Input: part model. Units: mm. Frame: model coordinates. A direction names the side the tool comes from. Give positions to 0.01 mm unless a question says otherwise; leave off trailing zeros. Order: outer loops, then holes, each group sorted by start corner. A loop starts at its lowest first (then second) coordinate and runs counter-clockwise, first axis right, second up. Notation, with made-up numbers: M 87.25,-25.5 L 104.25,-25.5 A20 cw 104.25,4.5 Z; hole C -12,5 d10. An arc over 180 degrees is marked long. Use a Markdown table: item, result.
Autodesk Fusion 360 part; units mm, degrees
sketch "Sketch1" plane through (0, 0, 0) normal (0, 0, 1) x (1, 0, 0)
  line L0 (-27.5, 5) -> (27.5, 5)
  line L1 (27.5, 5) -> (27.5, -5)
  line L2 (27.5, -5) -> (-27.5, -5)
  line L3 (-27.5, -5) -> (-27.5, 5)
  line L4 (-27.5, 5) -> (27.5, -5) construction
  line L5 (27.5, 5) -> (-27.5, -5) construction
  dimension "d1" = 55
  dimension "d2" = 10
sketch "Sketch2" plane through (0, 0, 0) normal (0, 0, 1) x (1, 0, 0)
  line L0 (-27.5, 0) -> (-20, 0) construction
  line L1 (27.5, 0) -> (20, 0) construction
  dimension "d3" = 7.5
  dimension "d4" = 7.5
sketch "Sketch3" plane through (0, 0, 0) normal (0, 0, 1) x (1, 0, 0)
  circle A0 centre (-20, 0) radius 1.8
  circle A1 centre (20, 0) radius 1.8
  dimension "d7" = 3.6
  dimension "d8" = 3.6
extrude "Extrude1" add sketch "Sketch1" along normal blind 2
extrude "Extrude2" cut sketch "Sketch3" along normal blind 10
sketch "Sketch5" plane through (0, 5, 0) normal (0, 1, 0) x (-1, 0, 0)
  line L0 (-27.5, 0) -> (27.5, 0)
  line L1 (27.5, 0) -> (27.5, 2)
  line L2 (27.5, 2) -> (-27.5, 2)
  line L3 (-27.5, 2) -> (-27.5, 0)
  line L4 (-5, 2) -> (5, 2)
  line L5 (5, 2) -> (5, 0)
  line L6 (5, 0) -> (-5, 0)
  line L7 (-5, 0) -> (-5, 2)
extrude "Extrude3" add sketch "Sketch5" along normal blind 25 contours L0 L2 L4 L5 L6 L7
sketch "Sketch6" plane through (0, 0, 2) normal (0, 0, 1) x (-1, 0, 0)
  circle A0 centre (-20, 0) radius 1.8
  circle A1 centre (20, 0) radius 1.8
  line L0 (27.5, 5) -> (-27.5, 5)
  line L1 (-27.5, 5) -> (-27.5, -5)
  line L2 (-27.5, -5) -> (-5, -5)
  line L3 (-5, -5) -> (-5, -30)
  line L4 (-5, -30) -> (5, -30)
  line L5 (5, -30) -> (5, -5)
  line L6 (5, -5) -> (27.5, -5)
  line L7 (27.5, -5) -> (27.5, 5)
  circle A2 centre (0, -25) radius 4.2426
extrude "Extrude4" add sketch "Sketch6" along normal blind 20 contours A2
fillet "Fillet1" radius 3 1 edges at (3.9555, 26.5342, 22)
fillet "Fillet2" radius 1 1 edges at (3.9555, 23.4658, 2)
chamfer "Chamfer1" distance 1 angle 45 8 edges at (-5, 17.5, 0) (5, 17.5, 0) (0, 30, 0) (-16.25, 5, 0) (-27.5, 0, 0) (0, -5, 0) (27.5, 0, 0) (16.25, 5, 0)
extrude "Extrude5" add 1 faces at (-5, 19.4745, 1.3333) along direction (-1, 0, 0) blind 5
extrude "Extrude6" add 1 faces at (5, 19.4745, 1.3333) along direction (1, 0, 0) blind 5
extrude "Extrude7" add 1 faces at (-0.5255, 30, 1.3333) along direction (0, 1, 0) blind 5
extrude "Extrude8" cut 1 faces at (1.6667, 35, 1.3333) along direction (0, -1, 0) blind 4
1) Material intervals for line 1 (X direction, y = 0, z = 1.2); line 2 (Y direction, x = -20, z = 1.5); line 3 (Z direction, x = -6.5, y = 22.5), sorted ascending. Write a range as from..to.
Response values:
| item | result |
|---|---|
| line 1 | x = -27.5..-21.8, -18.2..18.2, 21.8..27.5 |
| line 2 | y = -5..-1.8, 1.8..5 |
| line 3 | z = 1..2 |
2) Reachability of faces 4 (the face through (0, 25, 22)), 5 (the face through (-7, 18, 1)) from +Z, -Z, +X, -X, +Y, -Y: full face, straight path, thin tool, end or side. Return the list, or none.
Response values:
| item | result |
|---|---|
| face 4 | +Z, +X, -X, +Y, -Y |
| face 5 | -Z, +Y |
3) Mould query, pull axis Y, two halves, no side actions, for faces 1 (the face through (21.717, -0.541, 0.986)), 2 (the face through (0, 6, 0)), 3 (the face through (3, 22, 11)). Classes: released by +Y, released by -Y, zero draft, split by the parting line, or undercut.
Response values:
| item | result |
|---|---|
| face 1 | undercut |
| face 2 | zero draft |
| face 3 | split by the parting line |
4) Cut plane D-D on y = 14. Return loops of the section in (x, z), and give its area (3 significant figures).
Response values:
| item | result |
|---|---|
| outline | M -10,1 L -5,1 L -4,0 L 4,0 L 5,1 L 10,1 L 10,2 L -10,2 Z |
| area | 29.0 mm² |
5) Cut plane A-A on y = 0. Return loops of the section in (x, z).
Response values:
| item | result |
|---|---|
| outline | M -27.5,1 L -26.5,0 L -21.8,0 L -21.8,2 L -27.5,2 Z; M -18.2,0 L 18.2,0 L 18.2,2 L -18.2,2 Z; M 21.8,0 L 26.5,0 L 27.5,1 L 27.5,2 L 21.8,2 Z |
6) Cut plane B-B on x = 20. Return loops of the section in (y, z).
Response values:
| item | result |
|---|---|
| outline | M -5,1 L -4,0 L -1.8,0 L -1.8,2 L -5,2 Z; M 1.8,0 L 4,0 L 5,1 L 5,2 L 1.8,2 Z |
7) Cut plane C-C on x = 9. Return loops of the section in (y, z).
Response values:
| item | result |
|---|---|
| outline | M -5,1 L -4,0 L 4,0 L 5,1 L 31,1 L 31,2 L -5,2 Z |
8) First-contact query: pin 1 Ø1.1 at (y, z) = (24.5, 1.5) entering from -X; pin 2 Ø0.8 at (x, z) = (15, 1.5) entering from +Y; pin 3 Ø1 at (x, y) = (9, 19) entering from +Z; pin 4 Ø8 at (x, z) = (21.5, 9.5) entering from +Y. Flat tips, straight axial feed; report the tip coordinate or a pass-through.
Response values:
| item | result |
|---|---|
| pin 1 | stops at x = -10 |
| pin 2 | stops at y = 5 |
| pin 3 | stops at z = 2 |
| pin 4 | passes through |
